Design review of the part built by this model. Coordinates are the model's own, in mm. Coordinates: 2 decimals unless noted, no trailing zeros. Loops run counter-clockwise (first coordinate to the right, second up) from the corner with the lowest first, then second, coordinate; pieces in that order, holes last. Notation, with made-up numbers: (-33.5, -32) -> (23.5, -32) arc R17 ccw to (23.5, -14) -> close; hole circle Ø11 at (-29.75, -17). An arc over 180 degrees is marked (long way). Use one line per item in the form item = value. Start each with the question number.
1. Consider section D-D (z = -62.5). State the section outline as (x, y) points (3 decimals), then the cut area to 3 significant figures.
2. Consider section A-A (z = -114). State the section outline as (x, y) points (3 decimals), then the cut area to 3 significant figures.
3. For pin 1 (12 mm diameter, centred on x = -147.5, z = -49, fed in from -Y), flat-tipped, find the tip position at first contact; note if it passes through.
4. Consider section B-B (y = 1). State the section outline as (x, z) points.
5. Wall thickness on line 1 (X direction, y = 2, z = -96.5); line 2 (X direction, y = 0.75, z = -97); line 3 (Z direction, x = -122, y = 2.85): over which ranges is each line inside the solid? List them lowest first. Write a range as from..to.
6. Consider section C-C (x = -101.6). State the section outline as (y, z) points (3 decimals), then the cut area to 3 significant figures.
Autodesk Inventor part; units mm, degrees
ref_plane "YZ Plane" through (0, 0, 0) normal (1, 0, 0) x (0, 1, 0)
ref_plane "XZ Plane" through (0, 0, 0) normal (0, 1, 0) x (-1, 0, 0)
ref_plane "XY Plane" through (0, 0, 0) normal (0, 0, 1) x (1, 0, 0)
sketch "Sketch1" plane through (0, 0, 0) normal (0, 1, 0) x (-1, 0, 0)
  line L0 (0, 0) -> (203.2, 0)
  line L1 (203.2, 0) -> (203.2, -254)
  line L2 (203.2, -254) -> (0, -254)
  line L3 (0, -254) -> (0, 0)
  line L4 (203.2, -127) -> (0, -127)
  line L5 (101.6, -254) -> (101.6, 0)
  circle A0 centre (101.6, -127) radius 69.85
  point P0 (171.45, -127)
  point P1 (31.75, -127)
  dimension "d0" = 203.2
  dimension "d1" = 254
  dimension "d2" = 139.7
extrude "Extrusion1" add sketch "Sketch1" along normal blind 3.175 contours L0 L5 A0 L4 L3 | L0 L1 L4 A0 L5
properties part number "2 Bottom Frame Base 2"
Geometry check:
q1.outline = (-203.2, 0) -> (-128.41, 0) -> (-128.41, 3.175) -> (-203.2, 3.175) -> close; (-74.79, 0) -> (0, 0) -> (0, 3.175) -> (-74.79, 3.175) -> close
q1.area = 475 mm²
q2.outline = (-203.2, 0) -> (-170.23, 0) -> (-170.23, 3.175) -> (-203.2, 3.175) -> close; (-32.97, 0) -> (0, 0) -> (0, 3.175) -> (-32.97, 3.175) -> close
q2.area = 209 mm²
q3.pin_1 = 0
q4.outline = (-203.2, -127) -> (-171.45, -127) arc R69.85 cw to (-31.75, -127) -> (0, -127) -> (0, 0) -> (-203.2, 0) -> close
q5.line_1 = -203.2..-164.44, -38.76..0
q5.line_2 = -203.2..-164.68, -38.52..0
q5.line_3 = -60.2..0
q6.outline = (0, -57.15) -> (3.175, -57.15) -> (3.175, 0) -> (0, 0) -> close
q6.area = 181 mm²
